For this review, take the finished solid that the model builds, in its own axes (mm). Round coordinates to 2 decimals unless told otherwise and drop trailing zeros. Order: outer loops, then holes, each group sorted by start corner. A loop starts at its lowest first (then second) coordinate and runs counter-clockwise, first axis right, second up. Notation, with made-up numbers: (-15.5, 6) -> (32.5, 6) arc R19 ccw to (32.5, 31) -> close; hole circle Ø5 at (57, -37). An arc over 180 degrees is marked (long way). Put each result on its own line as item: value. Start each with the question number.
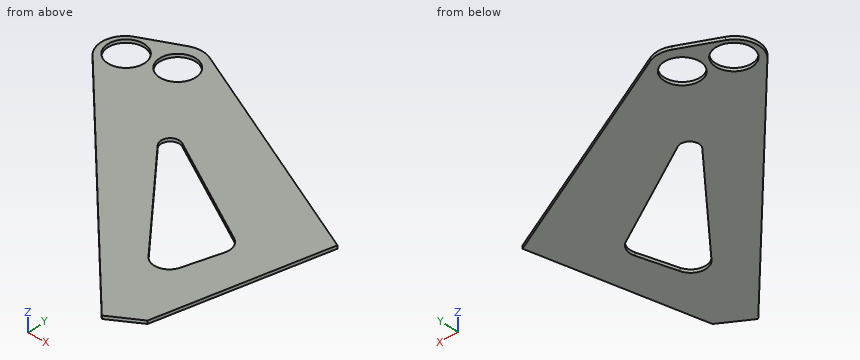
```python
from build123d import *

# Parameters (mm, degrees)
SKETCH_R   = 58.5
SKETCH_R_2 = 59.15
PAD_DEPTH  = 10


with BuildPart() as part:
    # Sketch → Pad (new body)
    with BuildSketch(Plane.XY):
        with BuildLine():
            Line((-424.386055, 871.427134), (318.446365, 91.122677))
            Line((318.446365, 91.122677), (413.307384, 149.460342))
            Line((413.307384, 149.460342), (538.173226, 685.49367))
            Line((538.173226, 685.49367), (-210.640671, 1052.542483))
            ThreePointArc((-210.640671, 1052.542483), (-245.83847, 1060.808988), (-281.126647, 1052.937227))
            Line((-281.126647, 1052.937227), (-401.436309, 995.626851))
            ThreePointArc((-401.436309, 995.626851), (-444.593461, 939.381275), (-424.386055, 871.427134))
        make_face()
        with Locations((-238.901588, 970.063171)):
            Circle(SKETCH_R, mode=Mode.SUBTRACT)
        with Locations((-369.619069, 930.28155)):
            Circle(SKETCH_R_2, mode=Mode.SUBTRACT)
        with BuildLine():
            ThreePointArc((-20.728661, 747.309936), (-58.68704, 740.721675), (-58.859603, 702.196177))
            Line((-58.859603, 702.196177), (236.819684, 345.945149))
            ThreePointArc((236.819684, 345.945149), (285.175775, 328.864216), (323.136202, 363.347195))
            Line((323.136202, 363.347195), (359.298187, 482.408455))
            ThreePointArc((359.298187, 482.408455), (357.97659, 515.265634), (336.53324, 540.196008))
            Line((-20.728661, 747.309936), (336.53324, 540.196008))
        make_face(mode=Mode.SUBTRACT)
    extrude(amount=PAD_DEPTH)


solid = part.part
```
Item 1: Consider section D-D, the plane x = -120. Write out the cut boundary in (y, z), plus the area to 3 significant figures.
Item 2: Consider section A-A, the plane x = 93. Write out the cut boundary in (y, z), plus the area to 3 significant figures.
Item 3: Consider section C-C, the plane z = 2.25. Write out the cut boundary in (x, y).
Item 4: Insertion check: pin 1 Ø1 at (x, z) = (-154, 3) entering from +Y; pin 2 Ø6 at (y, z) = (765.5, 3) entering from -X; pin 3 Ø2 at (y, z) = (271.5, 7.5) entering from -X. Each pin has a flat end and moves straight along its axis. Give the tip position at first contact, or say it passes through.
Item 5: Consider section B-B, the plane y = 588. Write out the cut boundary in (x, z), plus the area to 3 significant figures.
Item 6: For L1, parallel to X at y = 645.5, z = 7.25; L2, parallel to Y at x = -369, z = 8.5; L3, parallel to Y at x = -6, z = 4.5, list the stretches that pass through material, from the lowest coordinate up.
Evaluation:
1. outline: (551.69, 0) -> (1008.11, 0) -> (1008.11, 10) -> (551.69, 10) -> close
1. area: 4,560 mm^2
2. outline: (327.94, 0) -> (519.23, 0) -> (519.23, 10) -> (327.94, 10) -> close; (681.38, 0) -> (903.71, 0) -> (903.71, 10) -> (681.38, 10) -> close
2. area: 4,140 mm^2
3. outline: (-424.39, 871.43) -> (318.45, 91.12) -> (413.31, 149.46) -> (538.17, 685.49) -> (-210.64, 1052.54) arc R81 ccw to (-281.13, 1052.94) -> (-401.44, 995.63) arc R78 ccw to start; hole circle Ø118.3 at (-369.62, 930.28); hole circle Ø117 at (-238.9, 970.06); hole (-58.86, 702.2) -> (236.82, 345.95) arc R50 ccw to (323.14, 363.35) -> (359.3, 482.41) arc R50 ccw to (336.53, 540.2) -> (-20.73, 747.31) arc R30 ccw to start
4. pin 1: stops at y = 1025.02
4. pin 2: stops at x = -326.4
4. pin 3: stops at x = 145.78
5. outline: (-154.57, 0) -> (35.92, 0) -> (35.92, 10) -> (-154.57, 10) -> close; (254.07, 0) -> (515.46, 0) -> (515.46, 10) -> (254.07, 10) -> close
5. area: 4,520 mm^2
6. L1: x = -209.31 to -11.8, 154.89 to 528.86
6. L2: y = 813.25 to 871.13, 989.43 to 1011.08
6. L3: y = 431.94 to 638.51, 738.77 to 952.23
